For this review, take the finished solid that the model builds, in its own axes (mm). Face numbers are marked on the shaded views. A direction names the side the tool comes from. Coordinates: 2 decimals unless noted, no trailing zeros. Loops run counter-clockwise (first coordinate to the right, second up) from the corner with the lowest first, then second, coordinate; pieces in that order, holes last. Notation, with made-up numbers: (74, 71.5) - (114, 71.5) arc R15 cw to (114, 91.5) - close; hole circle Ø7 at (-9.75, -7.5). An arc over 180 degrees is marked (long way). One line per item, written item: value. Start each with the question number.
1. Take a section at A-A, the plane x = -63. State the section outline as (y, z) points, and give its area (3 significant figures).
2. For the marked faces 1, 2, 3 and 4, list the 3-axis set-ups (+Z, -Z, +X, -X, +Y, -Y) from which the entire face can be reached by the end or side of a thin tool; tool diameter is ignored.
3. The part is to be moulded in two halves that separate along X. For the marked faces 5, 6 and 7, say which applies: released by +X, released by -X, zero draft, split by the parting line, or undercut.
4. Take a section at D-D, the plane z = -7. State the section outline as (x, y) points.
5. To check wall thickness, follow line 1 (X direction, y = 4.5, z = -21); line 2 (X direction, y = -42, z = 20); line 3 (X direction, y = -52.25, z = -20). State the ranges of each line that lie inside material, in increasing order. Write a range as from..to.
6. Take a section at B-B, the plane y = -19.5. State the section outline as (x, z) points, and give its area (3 significant figures).
7. Insertion check: pin 1 (16 mm diameter, centred on x = -64, z = -8.5, fed in from +Y); pin 2 (10.5 mm diameter, centred on x = 63, z = 20, fed in from -Y); pin 3 (10.5 mm diameter, centred on x = -32, z = -21, fed in from -Y); pin 4 (12 mm diameter, centred on y = -32.5, z = -21, fed in from +X). Each pin has a flat end and moves straight along its axis. Give the tip position at first contact, or say it passes through.
8. Take a section at C-C, the plane x = 63. State the section outline as (y, z) points.
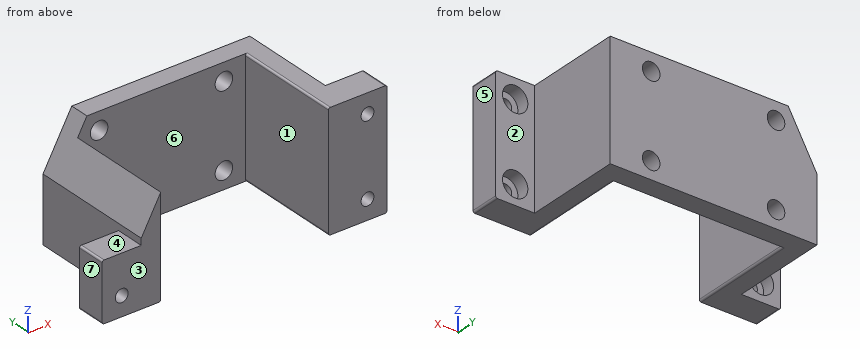
```python
from build123d import *

# Parameters (mm, degrees)
SKETCH1_W           = 106
SKETCH1_H           = 60
BOSS_EXTRUDE1_DEPTH = 10
SKETCH2_W           = 10
SKETCH2_H           = 60
BOSS_EXTRUDE2_DEPTH = 55
SKETCH3_W           = 60
SKETCH3_H           = 15
BOSS_EXTRUDE3_DEPTH = 20
SKETCH4_W           = 30
SKETCH4_H           = 15
BOSS_EXTRUDE4_DEPTH = 20
SKETCH5_R           = 4.5
CUT_EXTRUDE1_DEPTH  = 66
SKETCH6_R           = 6.5
CUT_EXTRUDE2_DEPTH  = 6.6
SKETCH7_R           = 3.3
CUT_EXTRUDE3_DEPTH  = 9.4
CUT_EXTRUDE4_DEPTH  = 66
FILLET1_R           = 1


with BuildPart() as part:
    # Sketch1 → Boss-Extrude1 (new body)
    with BuildSketch(Plane(origin=(0, 0, 0), x_dir=(1, 0, 0), z_dir=(0, 1, 0))):
        Rectangle(SKETCH1_W, SKETCH1_H)
    extrude(amount=BOSS_EXTRUDE1_DEPTH)

    # Sketch2 → Boss-Extrude2 (add)
    with BuildSketch(Plane.XZ):
        with Locations((-48, 0)):
            Rectangle(SKETCH2_W, SKETCH2_H)
        with Locations((48, 0)):
            Rectangle(SKETCH2_W, SKETCH2_H)
    extrude(amount=BOSS_EXTRUDE2_DEPTH)

    # Sketch3 → Boss-Extrude3 (add)
    with BuildSketch(Plane(origin=(53, 0, 0), x_dir=(0, 0, -1), z_dir=(1, 0, 0))):
        with Locations((0, -47.5)):
            Rectangle(SKETCH3_W, SKETCH3_H)
    extrude(amount=BOSS_EXTRUDE3_DEPTH)

    # Sketch4 → Boss-Extrude4 (add)
    with BuildSketch(Plane.ZY.offset(53)):
        with Locations((-15, -47.5)):
            Rectangle(SKETCH4_W, SKETCH4_H)
    extrude(amount=BOSS_EXTRUDE4_DEPTH)

    # Sketch5 → Cut-Extrude1 (cut, through all)
    with BuildSketch(Plane(origin=(0, 10, 0), x_dir=(1, 0, 0), z_dir=(0, 1, 0))):
        with Locations((-32, 21)):
            Circle(SKETCH5_R)
        with Locations((32, 21)):
            Circle(SKETCH5_R)
        with Locations((32, -21)):
            Circle(SKETCH5_R)
        with Locations((-32, -21)):
            Circle(SKETCH5_R)
    extrude(amount=-CUT_EXTRUDE1_DEPTH, mode=Mode.SUBTRACT)

    # Sketch6 → Cut-Extrude2 (cut)
    with BuildSketch(Plane(origin=(0, -40, 0), x_dir=(1, 0, 0), z_dir=(0, 1, 0))):
        with Locations((63, 20)):
            Circle(SKETCH6_R)
        with Locations((63, -20)):
            Circle(SKETCH6_R)
        with Locations((-63, 20)):
            Circle(SKETCH6_R)
    extrude(amount=-CUT_EXTRUDE2_DEPTH, mode=Mode.SUBTRACT)

    # Sketch7 → Cut-Extrude3 (cut, through all)
    with BuildSketch(Plane(origin=(0, -46.6, 0), x_dir=(1, 0, 0), z_dir=(0, 1, 0))):
        with Locations((-63, 20)):
            Circle(SKETCH7_R)
        with Locations((63, -20)):
            Circle(SKETCH7_R)
        with Locations((63, 20)):
            Circle(SKETCH7_R)
    extrude(amount=-CUT_EXTRUDE3_DEPTH, mode=Mode.SUBTRACT)

    # Sketch8 → Cut-Extrude4 (cut, through all)
    with BuildSketch(Plane(origin=(0, 10, 0), x_dir=(1, 0, 0), z_dir=(0, 1, 0))):
        Polygon((-38.239, -30), (-53, -3.370451084), (-53, -30), align=None)
    extrude(amount=-CUT_EXTRUDE4_DEPTH, mode=Mode.SUBTRACT)

    # Fillet1
    fillet1_edges = [part.edges().sort_by_distance(p)[0] for p in [
        (-43, -27.5, -30),
        (43, -27.5, 30),
        (43, -27.5, -30),
        (73, -47.5, 30),
        (73, -47.5, -30),
        (-73, -47.5, -30),
        (-73, -47.5, 0),
    ]]
    fillet(fillet1_edges, radius=FILLET1_R)


solid = part.part
```
Solutions:
1. outline: (-55, -30) - (-40, -30) - (-40, -26.5) - (-46.6, -26.5) - (-46.6, -23.3) - (-55, -23.3) - close; (-55, -16.7) - (-46.6, -16.7) - (-46.6, -13.5) - (-40, -13.5) - (-40, 0) - (-55, 0) - close
1. area: 309 mm2
2. face 1: +Z, -Z, -Y
2. face 2: +Z, -Z, +X, +Y
2. face 3: +Z, -Z, +X, -X, -Y
2. face 4: +Z, -X, +Y, -Y
3. face 5: released by +X
3. face 6: undercut
3. face 7: released by -X
4. outline: (-73, -55) - (-43, -55) - (-43, 0) - (43, 0) - (43, -55) - (73, -55) - (73, -40) - (53, -40) - (53, 10) - (-53, 10) - (-53, -40) - (-73, -40) - close
5. line 1: -53..-36.5, -27.5..27.5, 36.5..53
5. line 2: -43.78..-43, 43..56.5, 69.5..73
5. line 3: -73..-66.3, -59.7..-43, 43..59.7, 66.3..73
6. outline: (-53, -30) - (-44, -30) arc R1 ccw to (-43, -29) - (-43, 21.41) - (-53, 3.37) - close; (43, -29) arc R1 ccw to (44, -30) - (53, -30) - (53, 30) - (44, 30) arc R1 ccw to (43, 29) - close
6. area: 1,020 mm2
7. pin 1: y = -40
7. pin 2: y = -55
7. pin 3: y = 0
7. pin 4: x = 53
8. outline: (-55, -30) - (-40, -30) - (-40, -26.5) - (-46.6, -26.5) - (-46.6, -23.3) - (-55, -23.3) - close; (-55, -16.7) - (-46.6, -16.7) - (-46.6, -13.5) - (-40, -13.5) - (-40, 13.5) - (-46.6, 13.5) - (-46.6, 16.7) - (-55, 16.7) - close; (-55, 23.3) - (-46.6, 23.3) - (-46.6, 26.5) - (-40, 26.5) - (-40, 30) - (-55, 30) - close
